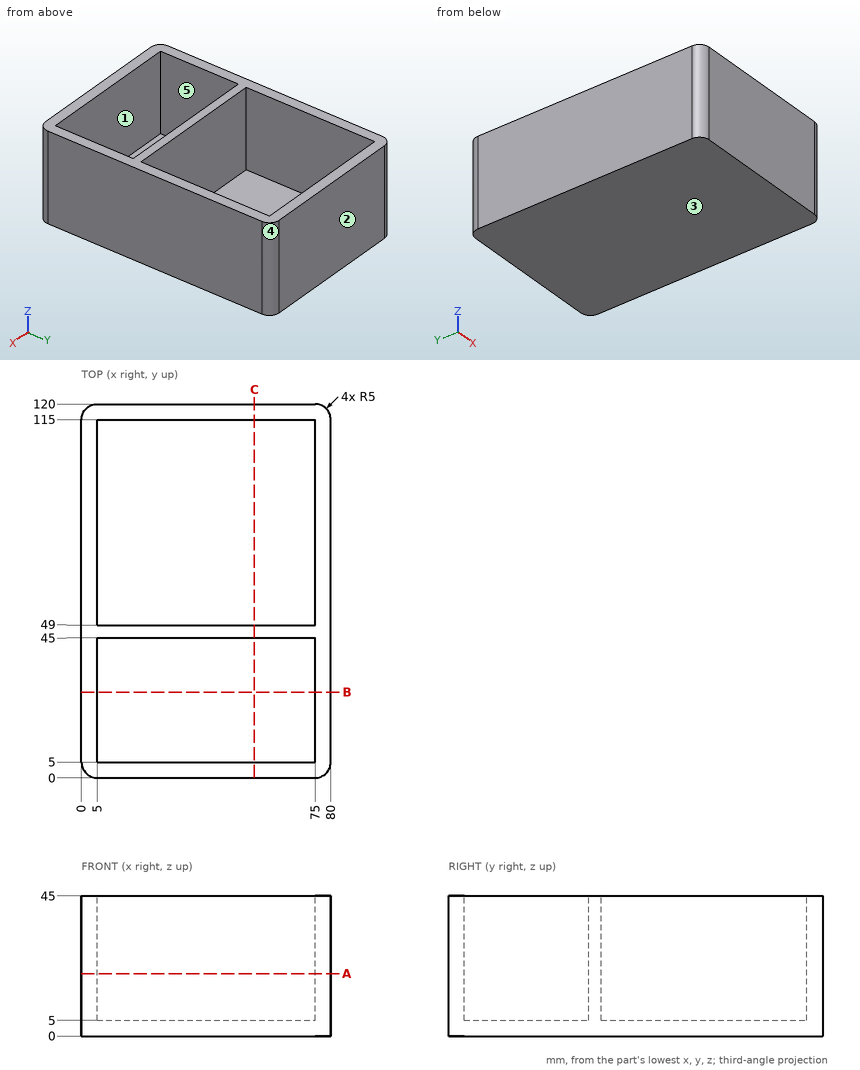
Design review of the part shown in the three views and the two pictorial views. Dimensions are in mm from the part's minimum x, y and z. A direction names the side the tool comes from. Round coordinates to 2 decimals unless told otherwise and drop trailing zeros. Write each loop counter-clockwise with the first axis right and the second up, starting at its lowest first coordinate (ties: lowest second). Pieces come first, ordered by that corner, then holes. Notation, with made-up numbers: (34, -8) -> (85, -8) arc R11 cw to (85, 6) -> close; hole circle Ø3 at (-38.75, 22.5). An arc over 180 degrees is marked (long way). One line per question, with ' | ' between items. Start each with the question number.
1) Add section C-C (x = 55.5). Write out the cut boundary in (y, z), and give its area (3 significant figures).
2) Add section A-A (z = 20). Write out the cut boundary in (x, y), and give its area (3 significant figures).
3) Add section B-B (y = 27.5). Write out the cut boundary in (x, z), and give its area (3 significant figures).
4) Wall thickness on line 1 along Y through (x, z) = (11.5, 23); line 2 along X through (y, z) = (35, 12); line 3 along Z through (x, y) = (41, 79.5): over which ranges is each line inside the solid? List them lowest first.
5) Machinability: for the marked faces 1 and 2, which of the approach directions +Z, -Z, +X, -X, +Y, -Y give a long, thin tool a straight path to every point of the face, cutting with its end or side? Answer none if there is none.
6) Mouldability with a two-part tool opening along Y and no side actions: class the marked faces 3, 4 and 5 as +Y half, -Y half, draft (parallel to the pull), parting line (faces both ways), or undercut.
Reported:
1) outline: (0, 0) -> (120, 0) -> (120, 45) -> (115, 45) -> (115, 5) -> (49, 5) -> (49, 45) -> (45, 45) -> (45, 5) -> (5, 5) -> (5, 45) -> (0, 45) -> close | area: 1,160 mm²
2) outline: (0, 5) arc R5 ccw to (5, 0) -> (75, 0) arc R5 ccw to (80, 5) -> (80, 115) arc R5 ccw to (75, 120) -> (5, 120) arc R5 ccw to (0, 115) -> close; hole (5, 5) -> (75, 5) -> (75, 45) -> (5, 45) -> close; hole (5, 49) -> (75, 49) -> (75, 115) -> (5, 115) -> close | area: 2,160 mm²
3) outline: (0, 0) -> (80, 0) -> (80, 45) -> (75, 45) -> (75, 5) -> (5, 5) -> (5, 45) -> (0, 45) -> close | area: 800 mm²
4) line 1: y = 0 to 5, 45 to 49, 115 to 120 | line 2: x = 0 to 5, 75 to 80 | line 3: z = 0 to 5
5) face 1: +Z | face 2: +Z, -Z, +X, -X, +Y
6) face 3: draft | face 4: +Y half | face 5: undercut
